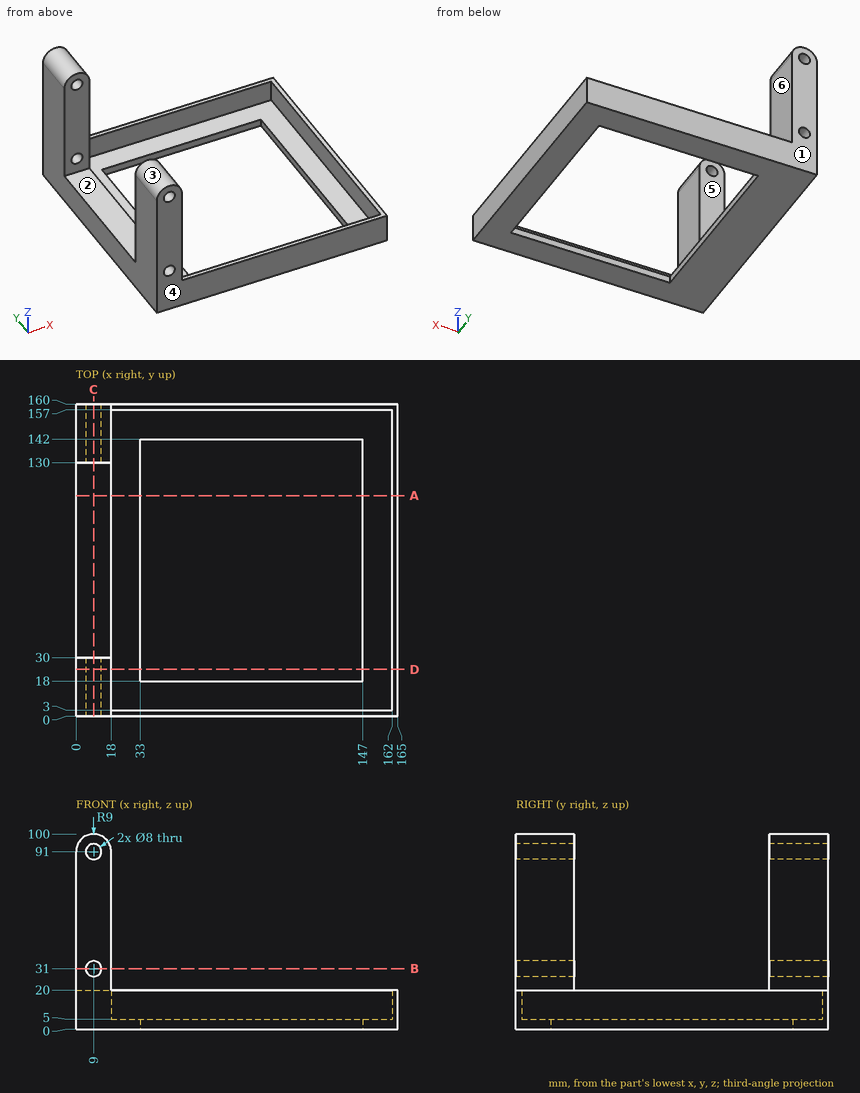
Part print with two shaded views. Sizes in mm from the minimum x, y, z corner. A direction names the side the tool comes from. Give positions to 0.01 mm unless a question says otherwise; leave off trailing zeros. Order: outer loops, then holes, each group sorted by start corner. A loop starts at its lowest first (then second) coordinate and runs counter-clockwise, first axis right, second up. Notation, with made-up numbers: (-9, -2.75) - (5, -2.75) arc R15 ccw to (5, 26.25) - close; hole circle Ø1 at (68.5, 88.5). An arc over 180 degrees is marked (long way). Write each question's results on one line, items separated by ' | '.
1. 3-axis set-ups, long thin cutter, end or side, ignore diameter. For the marked faces 4, 5 and 6: which of +Z, -Z, +X, -X, +Y, -Y reach the whole face in a straight line?
Calculated:
face 4: +Z, -Z, +X, -X, -Y | face 5: +Z, +X, -X | face 6: +Z
2. Saw through at D-D on y = 24. List the corners of the cut face in (x, z), and give its area (3 significant figures).
Calculated:
outline: (0, 0) - (33, 0) - (33, 5) - (18, 5) - (18, 91) arc R9 ccw to (0, 91) - close; (147, 0) - (165, 0) - (165, 20) - (162, 20) - (162, 5) - (147, 5) - close; hole circle Ø8 at (9, 31); hole circle Ø8 at (9, 91) | area: 1,870 mm2
3. Probe L1, parallel to Z at x = 9, y = 19; L2, parallel to X at y = 34.5, z = 7; L3, parallel to Y at x = 97, z = 7. List the from-to ranges inside material, lowest first. Write a range as from..to.
Calculated:
L1: z = 0..27, 35..87, 95..100 | L2: x = 0..18, 162..165 | L3: y = 0..3, 157..160
4. Saw through at B-B on z = 31. List the corners of the cut face in (x, y).
Calculated:
outline: (0, 0) - (5, 0) - (5, 30) - (0, 30) - close; (0, 130) - (5, 130) - (5, 160) - (0, 160) - close; (13, 0) - (18, 0) - (18, 30) - (13, 30) - close; (13, 130) - (18, 130) - (18, 160) - (13, 160) - close
5. Saw through at A-A on y = 113. List the corners of the cut face in (x, z), and give its area (3 significant figures).
Calculated:
outline: (0, 0) - (33, 0) - (33, 5) - (18, 5) - (18, 20) - (0, 20) - close; (147, 0) - (165, 0) - (165, 20) - (162, 20) - (162, 5) - (147, 5) - close | area: 570 mm2
6. Pull direction Y, two halves, no side cores. Call the marked faces 1, 2 and 3: released by +Y, released by -Y, zero draft, split by the parting line, or undercut.
Calculated:
face 1: released by +Y | face 2: undercut | face 3: zero draft
7. Pin check, flat tips, straight feed: pin 1 (9 mm diameter, centred on x = 5, y = 55, fed in from +Z); pin 2 (8 mm diameter, centred on y = 23.5, z = 48, fed in from +X). Stop position of each tip, or through.
Calculated:
pin 1: stops at z = 20 | pin 2: stops at x = 18
8. Saw through at C-C on x = 9. List the corners of the cut face in (y, z), and give its area (3 significant figures).
Calculated:
outline: (0, 0) - (160, 0) - (160, 27) - (130, 27) - (130, 20) - (30, 20) - (30, 27) - (0, 27) - close; (0, 35) - (30, 35) - (30, 87) - (0, 87) - close; (0, 95) - (30, 95) - (30, 100) - (0, 100) - close; (130, 35) - (160, 35) - (160, 87) - (130, 87) - close; (130, 95) - (160, 95) - (160, 100) - (130, 100) - close | area: 7,040 mm2
